Geometry check sheet. Reference: drawing and pictorial views, mm from the part's lowest x, y, z. A direction names the side the tool comes from. Coordinates: 2 decimals unless noted, no trailing zeros. Loops run counter-clockwise (first coordinate to the right, second up) from the corner with the lowest first, then second, coordinate; pieces in that order, holes last. Notation, with made-up numbers: (57.25, 60) - (96.25, 60) arc R25 cw to (96.25, 85) - close; hole circle Ø11 at (-12, 87.25). An arc over 180 degrees is marked (long way). One line per item, written item: value.
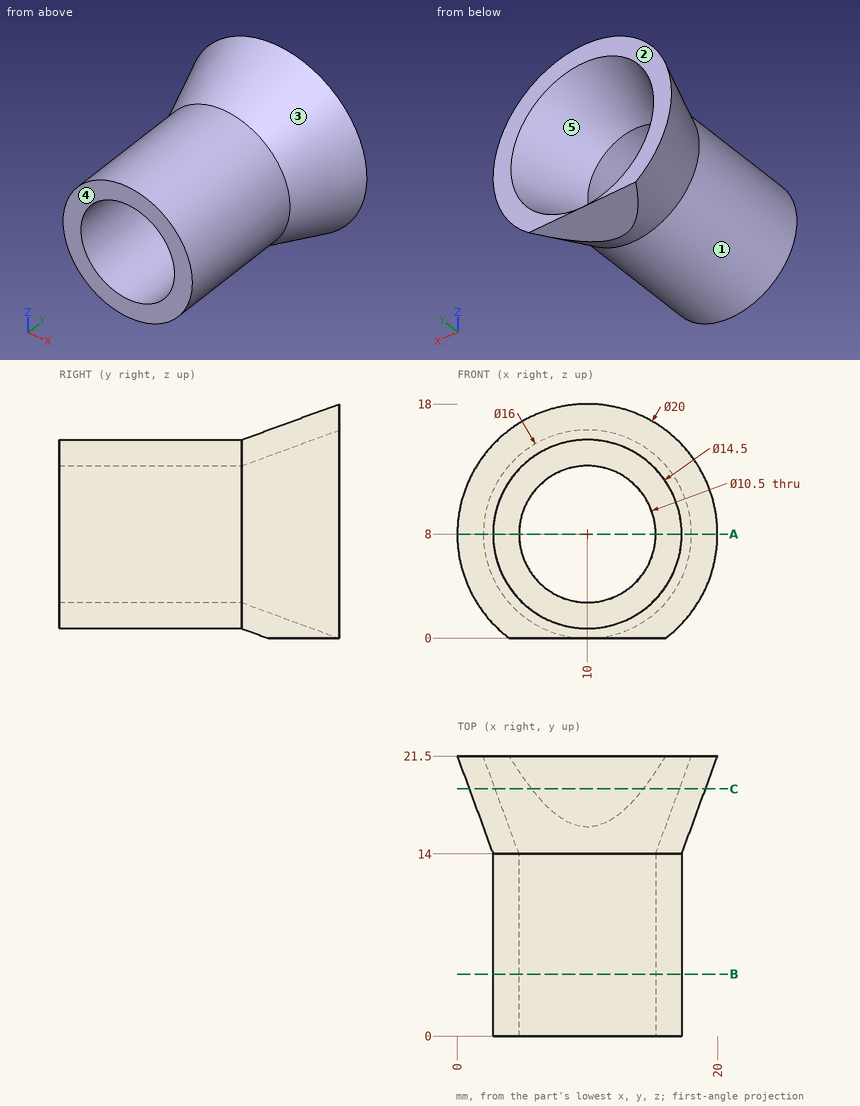
(1) Access from +Z, -Z, +X, -X, +Y, -Y to the whole of each face (thin tool, end or side, straight path). Record for the marked faces 1 and 2.
Reply:
face 1: -Y
face 2: +Z, -Z, +X, -X, +Y
(2) Cross-section at C-C on y = 19. Record the cut outline in (x, z), and give its area (3 significant figures).
Reply:
outline: (5.7, 0) - (14.3, 0) arc R9.08 ccw (long way) to start; hole circle Ø14.17 at (10, 8)
area: 95.3 mm2
(3) Material ranges on probe 1 along Z at (x, y) = (10, 6.75); probe 2 along Z at (x, y) = (10, 17.5); probe 3 along X at (y, z) = (1.25, 5.5), recorded low to high. Write a range as from..to.
Reply:
probe 1: 0.75..2.75, 13.25..15.25
probe 2: 0..1.47, 14.53..16.53
probe 3: 3.19..5.38, 14.62..16.81
(4) Cross-section at B-B on y = 4.75. Record the cut outline in (x, z), and give its area (3 significant figures).
Reply:
outline: circle Ø14.5 at (10, 8); hole circle Ø10.5 at (10, 8)
area: 78.5 mm2
(5) Cross-section at A-A on z = 8. Record the cut outline in (x, y), and give its area (3 significant figures).
Reply:
outline: (0, 21.5) - (2.75, 14) - (2.75, 0) - (4.75, 0) - (4.75, 14) - (2, 21.5) - close; (15.25, 0) - (17.25, 0) - (17.25, 14) - (20, 21.5) - (18, 21.5) - (15.25, 14) - close
area: 86.0 mm2
(6) Release check for a two-part mould opening along Z. For the marked faces 3, 4 and 5 record: pulls with the +Z half, pulls with the -Z half, needs draft (parallel to the pull), parting line crosses it, or undercut.
Reply:
face 3: parting line crosses it
face 4: needs draft
face 5: undercut
(7) Go/stop test with flat-tipped pins: pin 1 Ø3 at (x, y) = (7.5, 15) entering from -Z; pin 2 Ø5 at (x, y) = (17.5, 13.5) entering from -Z; pin 3 Ø5 at (x, y) = (4, 12) entering from +Z. Record where each tip stops, or that it passes through.
Reply:
pin 1: z = 0.1
pin 2: z = 2.69
pin 3: z = 14.35
